from build123d import *

# Parameters (mm, degrees)
F0_W     = 110.2
F0_H     = 60.2
F1_DEPTH = 3
F0_W_2   = 116.2
F0_H_2   = 66.2
F2_DEPTH = 9
F3_W     = 35.35
F3_H     = 6
F4_DEPTH = 1.5
F5_R     = 1.75
F6_DEPTH = 25
F5_R_2   = 2.75
F7_DEPTH = 1
F8_R     = 3


# Not quite as in the source:
# - a pattern or mirror of a feature is missing from the dataset's text; its kind, count and spacing are read off the source's solid


with BuildPart() as f1:
    # F0 (on Top) → F1 (new body)
    with BuildSketch(Plane.XY):
        Rectangle(F0_W, F0_H)
    extrude(amount=F1_DEPTH)

    # F0 (on Top) → F2 (join)
    with BuildSketch(Plane.XY):
        Rectangle(F0_W_2, F0_H_2)
        Rectangle(F0_W, F0_H, mode=Mode.SUBTRACT)
    extrude(amount=F2_DEPTH)

    # F3 (on face) → F4 (cut)
    with BuildSketch(Plane.XY.offset(3)):
        Polygon((-12.5, 10), (-12.5, 3), (-12.5, -3), (-12.5, -10), (12.5, -10), (12.5, -3), (12.5, 3), (12.5, 10), align=None)
        with Locations((-30.175, 0)):
            Rectangle(F3_W, F3_H)
        with Locations((30.175, 0)):
            Rectangle(F3_W, F3_H)
        Polygon((-47.85, 30.1), (-53.85, 30.1), (-53.85, -30.1), (-47.85, -30.1), (-47.85, -3), (-47.85, 3), align=None)
        Polygon((53.85, 30.1), (47.85, 30.1), (47.85, 3), (47.85, -3), (47.85, -30.1), (53.85, -30.1), align=None)
    extrude(amount=-F4_DEPTH, mode=Mode.SUBTRACT)

    # F5 (on face) → F6 (cut)
    with BuildSketch(Plane.XZ.offset(33.1)):
        with Locations((-50.85, 4.5)):
            Circle(F5_R)
        with Locations((50.85, 4.5)):
            Circle(F5_R)
    f6 = extrude(amount=-F6_DEPTH, mode=Mode.SUBTRACT)

    # F6_copies: F6 across plane
    add(f6.mirror(Plane.ZX), mode=Mode.SUBTRACT)

    # F5 (on face) → F7 (cut)
    with BuildSketch(Plane.XZ.offset(33.1)):
        with Locations((-50.85, 4.5)):
            Circle(F5_R_2)
        with Locations((-50.85, 4.5)):
            Circle(F5_R, mode=Mode.SUBTRACT)
        with Locations((-10, 4.5)):
            Circle(F5_R_2)
        with Locations((0, 4.5)):
            Circle(F5_R_2)
        with Locations((10, 4.5)):
            Circle(F5_R_2)
        with Locations((50.85, 4.5)):
            Circle(F5_R_2)
        with Locations((50.85, 4.5)):
            Circle(F5_R, mode=Mode.SUBTRACT)
    f7 = extrude(amount=-F7_DEPTH, mode=Mode.SUBTRACT)

    # F7_copies: F7 across plane
    add(f7.mirror(Plane.ZX), mode=Mode.SUBTRACT)

    # F8
    f8_edges = [f1.edges().sort_by_distance(p)[0] for p in [
        (58.1, -33.1, 4.5),
        (-58.1, -33.1, 4.5),
        (58.1, 33.1, 4.5),
        (-58.1, 33.1, 4.5),
    ]]
    fillet(f8_edges, radius=F8_R)


solid = f1.part
Build history of the part. All positions in model axes, mm. A direction names the side the tool comes from. Round coordinates to 2 decimals unless told otherwise and drop trailing zeros. Write each loop counter-clockwise with the first axis right and the second up, starting at its lowest first coordinate (ties: lowest second). Pieces come first, ordered by that corner, then holes. Notation, with made-up numbers: M -21.75,0.25 L 5.25,0.25 A21 cw 5.25,32.25 Z; hole C 41,45.5 d2. An arc over 180 degrees is marked long. Answer as a JSON object with one key per item and string values. Group by question number.
(1) Which spindle directions (+Z, -Z, +X, -X, +Y, -Y) get a long thin tool onto all of the face, cutting with end or side? Do faces 4 (the flat face through (-1, 30.1, 6)), 5 (the cylindrical face through (-48.31, 32.61, 3.45)), 6 (the flat face through (10, -32.1, 5)). Say none if no direction does.
(2) Drill centre lines: L1, parallel to Y at x = 10, z = 7; L2, parallel to Y at x = 19.5, z = 4.25; L3, parallel to X at y = 7.5, z = 6. Where is each one in solid material? Low to high.
(3) Cut at B-B (y = 24). Give the cut face in (x, z), and give its area (3 significant figures).
(4) Cut at D-D (z = 4.5). Give the number of separate pieces and of enclosed holes in the cut face, and give its area (3 significant figures).
(5) Mould opens along X. For faces 1 (the cylindrical face through (12.54, 32.61, 3.45)), 2 (the cylindrical face through (57.2, 32.24, 4.56)), 3 (the cylindrical face through (-57.24, 32.2, 4.56)) say: pulls with the +X half, pulls with the -X half, needs draft (parallel to the pull), parting line crosses it, or undercut.
(6) Cut at A-A (x = -50.85). Give the cut face in (y, z), and give its area (3 significant figures).
(7) Cut at C-C (x = 10). Give the cut face in (y, z).
(8) Flat gauge pins, fed straight in: pin 1 (5 mm diameter, centred on x = -17.5, y = 2.5, fed in from +Z); pin 2 (8 mm diameter, centred on x = 3, y = 5.5, fed in from +Z); pin 3 (4.5 mm diameter, centred on x = 10, z = 4.5, fed in from -Y). Where does each tip first touch, or does it go through?
Responses:
{
 "1": {"face 4": "+Z", "face 5": "+Y", "face 6": "-Y"},
 "2": {"L1": "y = -32.1 to -30.1, 30.1 to 32.1", "L2": "y = -33.1 to -30.1, 30.1 to 33.1", "L3": "x = -58.1 to -55.1, 55.1 to 58.1"},
 "3": {"outline": "M -58.1,0 L 58.1,0 L 58.1,9 L 55.1,9 L 55.1,3 L 53.85,3 L 53.85,1.5 L 47.85,1.5 L 47.85,3 L -47.85,3 L -47.85,1.5 L -53.85,1.5 L -53.85,3 L -55.1,3 L -55.1,9 L -58.1,9 Z", "area": "367 mm2"},
 "4": {"separate pieces": "4", "enclosed holes": "0", "area": "968 mm2"},
 "5": {"face 1": "undercut", "face 2": "pulls with the +X half", "face 3": "pulls with the -X half"},
 "6": {"outline": "M -33.1,0 L 33.1,0 L 33.1,1.75 L 32.1,1.75 L 32.1,2.75 L 30.1,2.75 L 30.1,1.5 L -30.1,1.5 L -30.1,2.75 L -32.1,2.75 L -32.1,1.75 L -33.1,1.75 Z; M -33.1,7.25 L -32.1,7.25 L -32.1,6.25 L -30.1,6.25 L -30.1,9 L -33.1,9 Z; M 30.1,6.25 L 32.1,6.25 L 32.1,7.25 L 33.1,7.25 L 33.1,9 L 30.1,9 Z", "area": "119 mm2"},
 "7": {"outline": "M -33.1,0 L 33.1,0 L 33.1,1.75 L 32.1,1.75 L 32.1,7.25 L 33.1,7.25 L 33.1,9 L 30.1,9 L 30.1,3 L 10,3 L 10,1.5 L -10,1.5 L -10,3 L -30.1,3 L -30.1,9 L -33.1,9 L -33.1,7.25 L -32.1,7.25 L -32.1,1.75 L -33.1,1.75 Z"},
 "8": {"pin 1": "stops at z = 3", "pin 2": "stops at z = 1.5", "pin 3": "stops at y = -32.1"}
}
